Autodesk Inventor part; units mm, degrees
ref_plane "YZ Plane" through (0, 0, 0) normal (1, 0, 0) x (0, 1, 0)
ref_plane "XZ Plane" through (0, 0, 0) normal (0, 1, 0) x (-1, 0, 0)
ref_plane "XY Plane" through (0, 0, 0) normal (0, 0, 1) x (1, 0, 0)
sketch "Sketch1" plane through (0, 0, 0) normal (0, 1, 0) x (-1, 0, 0)
  line L0 (-51.9938, 0) -> (-51.9938, 51.9938)
  line L1 (-51.9938, 51.9938) -> (0, 51.9938)
  line L2 (51.9938, 0) -> (51.9938, -51.9938)
  line L3 (51.9938, -51.9938) -> (0, -51.9938)
  line L4 (-51.9938, 0) -> (-51.9938, 51.9938)
  line L5 (-51.9938, 51.9938) -> (0, 51.9938)
  line L6 (-51.9938, 0) -> (-51.9938, -51.9938)
  line L7 (-51.9938, -51.9938) -> (0, -51.9938)
  line L8 (51.9938, 0) -> (51.9938, 51.9938)
  line L9 (51.9938, 51.9938) -> (0, 51.9938)
  point P0 (0, 0)
  dimension "d0" = 51.9938
  dimension "d1" = 51.9938
  dimension "d2" = 51.9938
  dimension "d3" = 51.9938
  dimension "d4" = 51.9938
  dimension "d5" = 51.9938
  dimension "d6" = 51.9938
  dimension "d7" = 51.9938
  dimension "d8" = 51.9938
  dimension "d9" = 51.9938
extrude "Extrusion1" add sketch "Sketch1" against normal blind 3
sketch "Sketch2" plane through (0, 0, 0) normal (0, 1, 0) x (1, 0, 0)
  line L0 (54.991, 0) -> (54.991, -54.991)
  line L1 (54.991, -54.991) -> (0, -54.991)
  line L2 (-54.991, 0) -> (-54.991, -54.991)
  line L3 (-54.991, -54.991) -> (0, -54.991)
  line L4 (-54.991, 0) -> (-54.991, 54.991)
  line L5 (-54.991, 54.991) -> (0, 54.991)
  line L6 (54.991, 0) -> (54.991, 54.991)
  line L7 (54.991, 54.991) -> (0, 54.991)
  line L8 (-51.9938, 51.9938) -> (51.9938, 51.9938)
  line L9 (51.9938, 0) -> (51.9938, 51.9938)
  line L10 (51.9938, 51.9938) -> (0, 51.9938)
  line L11 (51.9938, 0) -> (51.9938, -51.9938)
  line L12 (51.9938, -51.9938) -> (0, -51.9938)
  line L13 (-51.9938, 0) -> (-51.9938, -51.9938)
  line L14 (-51.9938, -51.9938) -> (0, -51.9938)
  line L15 (-51.9938, 0) -> (-51.9938, 51.9938)
  line L16 (-51.9938, 51.9938) -> (0, 51.9938)
  point P0 (0, 0)
  dimension "d14" = 54.991
  dimension "d15" = 54.991
  dimension "d16" = 54.991
  dimension "d17" = 54.991
  dimension "d18" = 54.991
  dimension "d19" = 54.991
  dimension "d20" = 51.9938
  dimension "d21" = 51.9938
  dimension "d22" = 51.9938
  dimension "d23" = 51.9938
  dimension "d24" = 51.9938
  dimension "d25" = 51.9938
  dimension "d26" = 51.9938
  dimension "d27" = 51.9938
extrude "Extrusion2" add sketch "Sketch2" along normal blind 70 and the other way blind 3
sketch "Sketch3" plane through (0, -3, 0) normal (0, -1, 0) x (1, 0, 0)
  circle A0 centre (0, 0) radius 50.4952
  dimension "d32" = 100.9904
extrude "Extrusion3" add sketch "Sketch3" along normal blind 18
sketch "Sketch4" plane through (0, -21, 0) normal (0, -1, 0) x (1, 0, 0)
  circle A0 centre (0, 0) radius 30
  dimension "d35" = 60
extrude "Extrusion4" add sketch "Sketch4" along normal blind 90
sketch "Sketch6" plane through (0, -111, 0) normal (0, -1, 0) x (1, 0, 0)
  circle A0 centre (0, 0) radius 27.4955
  dimension "d39" = 54.991
hole "Hole1" at (0, -111, 0) direction (0, 1, 0) diameter 54.991 depth 111
chamfer "Chamfer1" distance 20.49 distance2 18 1 edges at (-50.4952, -21, 0) measured on face at (-21.4731, -21, -37.7754)
chamfer "Chamfer2" distance 17 distance2 18 1 edges at (0, 0, 27.4955) measured on face at (-43.7609, 0, -1.1047)
properties part number "PMT housing"
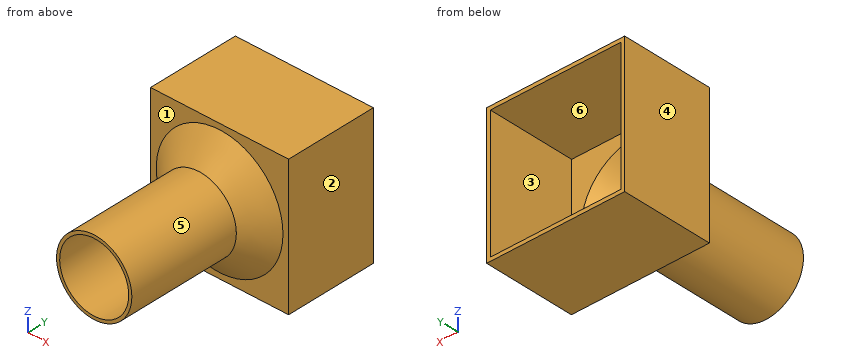
Geometry check sheet. Reference: the model listing, model coordinates, mm. Face numbers are marked on the shaded views. A direction names the side the tool comes from. Round coordinates to 2 decimals unless told otherwise and drop trailing zeros. Order: outer loops, then holes, each group sorted by start corner. A loop starts at its lowest first (then second) coordinate and runs counter-clockwise, first axis right, second up. Notation, with made-up numbers: (85, 86) - (106, 86) arc R17 ccw to (106, 94) - close; hole circle Ø9 at (9, -20.75). An arc over 180 degrees is marked (long way). One line per question, with ' | ' between items. Start each with the question number.
(1) Thickness scan on L1, parallel to Z at x = 0, y = -51; L2, parallel to X at y = 16, z = -4.5. Record the ranges inside material, lowest first. Write a range as [from, to].
(2) Depth check by flat-ended pin: pin 1 Ø6 at (x, y) = (25, -52.5) entering from -Z; pin 2 Ø3 at (y, z) = (-37, 27.5) entering from +X; pin 3 Ø3 at (x, y) = (-22, -13) entering from +Z. Enter the tip coordinate at first touch or a pass-through.
(3) Sectioned sample at C-C on y = -30. Record the cut outline in (x, z).
(4) Access from +Z, -Z, +X, -X, +Y, -Y to the whole of each face (thin tool, end or side, straight path). Record for the marked faces 1, 2 and 3.
(5) Release check for a two-part mould opening along Z. For the marked faces 4, 5 and 6 record: released by +Z, released by -Z, zero draft, split by the parting line, or undercut.
Conclusion:
1) L1: z = [-30, -27.5], [27.5, 30] | L2: x = [-54.99, -51.99], [51.99, 54.99]
2) pin 1: stops at z = -20.4 | pin 2: stops at x = 14.97 | pin 3: stops at z = 34.59
3) outline: circle Ø60 at (0, 0); hole circle Ø54.99 at (0, 0)
4) face 1: -Y | face 2: +Z, -Z, +X, +Y, -Y | face 3: +Y
5) face 4: zero draft | face 5: split by the parting line | face 6: undercut
